```python
from build123d import *

# Parameters (mm, degrees)
SKETCH1_W           = 23.16
SKETCH1_H           = 8.62
SKETCH1_R           = 1.75
BOSS_EXTRUDE1_DEPTH = 4
FILLET1_R           = 4


with BuildPart() as part:
    # Sketch1 → Boss-Extrude1 (new body)
    with BuildSketch(Plane.XY):
        Rectangle(SKETCH1_W, SKETCH1_H)
        with Locations((-7.85, 0)):
            Circle(SKETCH1_R, mode=Mode.SUBTRACT)
        with Locations((7.85, 0)):
            Circle(SKETCH1_R, mode=Mode.SUBTRACT)
        Circle(SKETCH1_R, mode=Mode.SUBTRACT)
    extrude(amount=BOSS_EXTRUDE1_DEPTH)

    # Fillet1
    fillet1_edges = [part.edges().sort_by_distance(p)[0] for p in [
        (11.58, -4.31, 2),
        (-11.58, -4.31, 2),
        (-11.58, 4.31, 2),
        (11.58, 4.31, 2),
    ]]
    fillet(fillet1_edges, radius=FILLET1_R)


solid = part.part
```
The model under review builds one solid part; all positions refer to its coordinate system, in mm. Give positions to 0.01 mm unless a question says otherwise; leave off trailing zeros. Write each loop counter-clockwise with the first axis right and the second up, starting at its lowest first coordinate (ties: lowest second). Pieces come first, ordered by that corner, then holes. Notation, with made-up numbers: (-22.5, 52.5) -> (-17.5, 52.5) arc R23 ccw to (-17.5, 69.5) -> close; hole circle Ø9 at (86, 38). An arc over 180 degrees is marked (long way). Put each result on its own line as item: value.
(1) We need section A-A, the plane x = 0. Give the boundary of the cut face in (y, z).
Results are:
outline: (-4.31, 0) -> (-1.75, 0) -> (-1.75, 4) -> (-4.31, 4) -> close; (1.75, 0) -> (4.31, 0) -> (4.31, 4) -> (1.75, 4) -> close
(2) For pin 1 Ø2 at (y, z) = (-2, 2.5) entering from +X; pin 2 Ø4 at (x, y) = (7.85, 0) entering from -Z, all flat-tipped, find the tip position at first contact; note any pin that passes through.
Results are:
pin 1: x = 11.52
pin 2: z = 0
(3) We need section D-D, the plane x = -7.85. Give the boundary of the cut face in (y, z), and give its area (3 significant figures).
Results are:
outline: (-4.3, 0) -> (-1.75, 0) -> (-1.75, 4) -> (-4.3, 4) -> close; (1.75, 0) -> (4.3, 0) -> (4.3, 4) -> (1.75, 4) -> close
area: 20.4 mm²
(4) To check wall thickness, follow probe 1 along X at (y, z) = (-0.25, 3.1); probe 2 along X at (y, z) = (-1.5, 1.6); probe 3 along Y at (x, z) = (-1.5, 3.55). State the ranges of each line that lie inside material, in increasing order. Write a range as from..to.
Results are:
probe 1: -11.58..-9.58, -6.12..-1.73, 1.73..6.12, 9.58..11.58
probe 2: -11.4..-8.75, -6.95..-0.9, 0.9..6.95, 8.75..11.4
probe 3: -4.31..-0.9, 0.9..4.31
(5) We need section B-B, the plane z = 0.7. Give the boundary of the cut face in (x, y).
Results are:
outline: (-11.58, -0.31) arc R4 ccw to (-7.58, -4.31) -> (7.58, -4.31) arc R4 ccw to (11.58, -0.31) -> (11.58, 0.31) arc R4 ccw to (7.58, 4.31) -> (-7.58, 4.31) arc R4 ccw to (-11.58, 0.31) -> close; hole circle Ø3.5 at (-7.85, 0); hole circle Ø3.5 at (0, 0); hole circle Ø3.5 at (7.85, 0)
(6) The part is to be moulded in two halves that separate along Y. For faces 1 (the flat face through (0, 4.31, 2)), 2 (the flat face through (0, 2, 4)), 3 (the cylindrical face through (6.1, 0.08, 1.97)), say which applies: pulls with the +Y half, pulls with the -Y half, needs draft (parallel to the pull), parting line crosses it, or undercut.
Results are:
face 1: pulls with the +Y half
face 2: needs draft
face 3: undercut
(7) We need section C-C, the plane y = 2.25. Give the boundary of the cut face in (x, z), and give its area (3 significant figures).
Results are:
outline: (-11.08, 0) -> (11.08, 0) -> (11.08, 4) -> (-11.08, 4) -> close
area: 88.6 mm²
